Part model, mm, in its own coordinate system. A direction names the side the tool comes from. Round coordinates to 2 decimals unless told otherwise and drop trailing zeros. Loops run counter-clockwise (first coordinate to the right, second up) from the corner with the lowest first, then second, coordinate; pieces in that order, holes last.
1) Drop flat-ended pins along their axis: P1, Ø0.6, axis at x = 26, y = 0, coming from the +Z side; P2, Ø1.5, axis at x = -12.5, y = 1, coming from the +Z side. Give the stop position or say it passes through.
2) Band-saw the part on B-B, the plane z = -17.5. Write the cut outline in (x, y).
3) Mould opens along X. For faces 1 (the cylindrical face through (13.92, 1.48, 35.59)), 2 (the flat face through (-0.032, 1.812, -13.179)), 3 (the cylindrical face through (-10.601, 1.479, -3.964)), 4 (the flat face through (-3, 3, -3)) say: +X half, -X half, draft (parallel to the pull), parting line (faces both ways), or undercut.
4) 3-axis set-ups, long thin cutter, end or side, ignore diameter. For faces 5 (the flat face through (0.032, 1.812, 13.179)), 6 (the flat face through (13, 1, -10)), 7 (the flat face through (-10, 1, -13)), 8 (the flat face through (-13, 1, 10)): which of +Z, -Z, +X, -X, +Y, -Y reach the whole face in a straight line?
5) Band-saw the part on A-A, the plane y = 1.25. Write the cut outline in (x, z), then the cut area to 3 significant figures.
6) Band-saw the part on D-D, the plane z = -36. Write the cut outline in (x, y).
7) Band-saw the part on C-C, the plane x = -5.5. Write the cut outline in (y, z).
8) Probe line 1 (Z direction, x = 0, y = 2.3); line 2 (Z direction, x = -28.5, y = 2.1); line 3 (Z direction, x = -22, y = 2.5). List the from-to ranges inside material, lowest first.
from build123d import *

# Parameters (mm, degrees)
F0_R     = 3.75
F1_DEPTH = 5
F3_DEPTH = 3
F4_R     = 55.5278104075
F5_DEPTH = 5
F6_R     = 2.5
F7_R     = 4
F8_DEPTH = 3.0010001


with BuildPart() as f1:
    # F0 (on Front) → F1 (new body)
    with BuildSketch(Plane.XZ):
        with BuildLine():
            Line((10, 7.379066267), (10, 18.8196601125))
            ThreePointArc((10, 18.8196601125), (14.0125853844, 35.3523313466), (0, 45))
            Line((0, 45), (0, 43))
            ThreePointArc((0, 43), (11.7683072321, 35.5233092337), (10, 21.6933761371))
            Line((10, 21.6933761371), (0, 13.1515390832))
            Line((0, 13.1515390832), (-0.8841328604, 12.3963272004))
            ThreePointArc((-0.8841328604, 12.3963272004), (-3.9176162816, 10.618189727), (-7.379066267, 10))
            Line((-7.379066267, 10), (-18.8196601125, 10))
            ThreePointArc((-18.8196601125, 10), (-35.3523313466, 14.0125853844), (-45, 0))
            Line((-45, 0), (-43, 0))
            ThreePointArc((-43, 0), (-35.5233092337, 11.7683072321), (-21.6933761371, 10))
            Line((-21.6933761371, 10), (-12.3963272004, -0.8841328604))
            ThreePointArc((-12.3963272004, -0.8841328604), (-10.618189727, -3.9176162816), (-10, -7.379066267))
            Line((-10, -7.379066267), (-10, -18.8196601125))
            ThreePointArc((-10, -18.8196601125), (-14.0125853844, -35.3523313466), (0, -45))
            Line((0, -45), (0, -43))
            ThreePointArc((0, -43), (-11.7683072321, -35.5233092337), (-10, -21.6933761371))
            Line((-10, -21.6933761371), (0.8841328604, -12.3963272004))
            ThreePointArc((0.8841328604, -12.3963272004), (3.9176162816, -10.618189727), (7.379066267, -10))
            Line((7.379066267, -10), (18.8196601125, -10))
            ThreePointArc((18.8196601125, -10), (35.3523313466, -14.0125853844), (45, 0))
            Line((45, 0), (43, 0))
            ThreePointArc((43, 0), (35.5233092337, -11.7683072321), (21.6933761371, -10))
            Line((21.6933761371, -10), (12.3963272004, 0.8841328604))
            ThreePointArc((12.3963272004, 0.8841328604), (10.618189727, 3.9176162816), (10, 7.379066267))
        make_face()
        Circle(F0_R, mode=Mode.SUBTRACT)
    extrude(amount=F1_DEPTH)

    # F2 (on face) → F3 (join)
    with BuildSketch(Plane(origin=(0, 0, 0), x_dir=(-1, 0, 0), z_dir=(0, 1, 0))):
        with BuildLine():
            Line((0, 43), (0, 45))
            ThreePointArc((0, 45), (-14.0125853844, 35.3523313466), (-10, 18.8196601125))
            Line((-10, 18.8196601125), (-10, 7.379066267))
            ThreePointArc((-10, 7.379066267), (-10.618189727, 3.9176162816), (-12.3963272004, 0.8841328604))
            Line((-12.3963272004, 0.8841328604), (-13.1515390832, 0))
            Line((-13.1515390832, 0), (-9.8753882025, 0))
            Line((-9.8753882025, 0), (-3.75, 0))
            ThreePointArc((-3.75, 0), (-2.6516504294, 2.6516504294), (0, 3.75))
            Line((0, 3.75), (0, 9.8753882025))
            Line((0, 9.8753882025), (0, 13.1515390832))
            Line((0, 13.1515390832), (-10, 21.6933761371))
            ThreePointArc((-10, 21.6933761371), (-11.7683072321, 35.5233092337), (0, 43))
        make_face()
        with BuildLine():
            Line((0, 13.1515390832), (0, 43))
            ThreePointArc((0, 43), (-11.7683072321, 35.5233092337), (-10, 21.6933761371))
            Line((-10, 21.6933761371), (0, 13.1515390832))
        make_face()
        with BuildLine():
            Line((0.8841328604, 12.3963272004), (0, 13.1515390832))
            Line((0, 13.1515390832), (0, 9.8753882025))
            Line((0, 9.8753882025), (0, 3.75))
            ThreePointArc((0, 3.75), (2.6516504294, 2.6516504294), (3.75, 0))
            Line((3.75, 0), (9.8753882025, 0))
            Line((9.8753882025, 0), (13.1515390832, 0))
            Line((13.1515390832, 0), (21.6933761371, 10))
            ThreePointArc((21.6933761371, 10), (35.5233092337, 11.7683072321), (43, 0))
            Line((43, 0), (45, 0))
            ThreePointArc((45, 0), (35.3523313466, 14.0125853844), (18.8196601125, 10))
            Line((18.8196601125, 10), (7.379066267, 10))
            ThreePointArc((7.379066267, 10), (3.9176162816, 10.618189727), (0.8841328604, 12.3963272004))
        make_face()
        with BuildLine():
            Line((-21.6933761371, -10), (-13.1515390832, 0))
            Line((-13.1515390832, 0), (-43, 0))
            ThreePointArc((-43, 0), (-35.5233092337, -11.7683072321), (-21.6933761371, -10))
        make_face()
        with BuildLine():
            Line((-9.8753882025, 0), (-13.1515390832, 0))
            Line((-13.1515390832, 0), (-21.6933761371, -10))
            ThreePointArc((-21.6933761371, -10), (-35.5233092337, -11.7683072321), (-43, 0))
            Line((-43, 0), (-45, 0))
            ThreePointArc((-45, 0), (-35.3523313466, -14.0125853844), (-18.8196601125, -10))
            Line((-18.8196601125, -10), (-7.379066267, -10))
            ThreePointArc((-7.379066267, -10), (-3.9176162816, -10.618189727), (-0.8841328604, -12.3963272004))
            Line((-0.8841328604, -12.3963272004), (0, -13.1515390832))
            Line((0, -13.1515390832), (0, -9.8753882025))
            Line((0, -9.8753882025), (0, -3.75))
            ThreePointArc((0, -3.75), (-2.6516504294, -2.6516504294), (-3.75, 0))
            Line((-3.75, 0), (-9.8753882025, 0))
        make_face()
        with BuildLine():
            ThreePointArc((3.75, 0), (2.6516504294, 2.6516504294), (0, 3.75))
            ThreePointArc((0, 3.75), (-2.6516504294, 2.6516504294), (-3.75, 0))
            ThreePointArc((-3.75, 0), (-2.6516504294, -2.6516504294), (0, -3.75))
            ThreePointArc((0, -3.75), (2.6516504294, -2.6516504294), (3.75, 0))
        make_face()
        with BuildLine():
            Line((9.8753882025, 0), (3.75, 0))
            ThreePointArc((3.75, 0), (2.6516504294, -2.6516504294), (0, -3.75))
            Line((0, -3.75), (0, -9.8753882025))
            Line((0, -9.8753882025), (0, -13.1515390832))
            Line((0, -13.1515390832), (10, -21.6933761371))
            ThreePointArc((10, -21.6933761371), (11.7683072321, -35.5233092337), (0, -43))
            Line((0, -43), (0, -45))
            ThreePointArc((0, -45), (14.0125853844, -35.3523313466), (10, -18.8196601125))
            Line((10, -18.8196601125), (10, -7.379066267))
            ThreePointArc((10, -7.379066267), (10.618189727, -3.9176162816), (12.3963272004, -0.8841328604))
            Line((12.3963272004, -0.8841328604), (13.1515390832, 0))
            Line((13.1515390832, 0), (9.8753882025, 0))
        make_face()
        with BuildLine():
            Line((21.6933761371, 10), (13.1515390832, 0))
            Line((13.1515390832, 0), (43, 0))
            ThreePointArc((43, 0), (35.5233092337, 11.7683072321), (21.6933761371, 10))
        make_face()
        with BuildLine():
            Line((10, -21.6933761371), (0, -13.1515390832))
            Line((0, -13.1515390832), (0, -43))
            ThreePointArc((0, -43), (11.7683072321, -35.5233092337), (10, -21.6933761371))
        make_face()
    extrude(amount=F3_DEPTH)

    # F4 (on face) → F5 (cut)
    with BuildSketch(Plane.XZ.offset(5)):
        Circle(F4_R)
    extrude(amount=-F5_DEPTH, mode=Mode.SUBTRACT)

    # F6
    f6_edges = [f1.edges().sort_by_distance(p)[0] for p in [
        (29.07577, 3, 0),
        (0, 3, 29.07577),
        (-29.07577, 3, 0),
        (0, 3, -29.07577),
    ]]
    fillet(f6_edges, radius=F6_R)

    # F7 (on face) → F8 (cut, through all)
    with BuildSketch(Plane.XZ):
        Circle(F7_R)
    extrude(amount=-F8_DEPTH, mode=Mode.SUBTRACT)


solid = f1.part
Reported:
1. P1: stops at z = 0
1. P2: stops at z = 10
2. outline: (-10, 0) - (0, 0) - (0, 0.5) arc R2.5 ccw to (-2.5, 3) - (-10, 3) - close
3. face 1: +X half
3. face 2: undercut
3. face 3: -X half
3. face 4: draft
4. face 5: +Z, +Y
4. face 6: -Z, +Y, -Y
4. face 7: -X, +Y, -Y
4. face 8: +Z, +Y, -Y
5. outline: (-45, 0.12) - (-13.25, 0.12) - (-12.4, -0.88) arc R10 cw to (-10, -7.38) - (-10, -18.82) arc R15 ccw to (-0.12, -45) - (-0.12, -13.25) - (0.88, -12.4) arc R10 cw to (7.38, -10) - (18.82, -10) arc R15 ccw to (45, -0.12) - (13.25, -0.12) - (12.4, 0.88) arc R10 cw to (10, 7.38) - (10, 18.82) arc R15 ccw to (0.12, 45) - (0.12, 13.25) - (-0.88, 12.4) arc R10 cw to (-7.38, 10) - (-18.82, 10) arc R15 ccw to start; hole circle Ø8 at (0, 0)
5. area: 2,030 mm2
6. outline: (-13.75, 0) - (0, 0) - (0, 0.5) arc R2.5 ccw to (-2.5, 3) - (-13.75, 3) - close
7. outline: (0, -43.96) - (3, -43.96) - (3, 10.18) - (0, 10.18) - close
8. line 1: z = -13.15 to -4, 4 to 13.15
8. line 2: z = 0.58 to 14.92
8. line 3: z = 1 to 12.69
